For this review, use the dimensioned drawing (mm, ordinates from the lowest corner) and the shaded views. A direction names the side the tool comes from. Coordinates: 2 decimals unless noted, no trailing zeros. Order: outer loops, then holes, each group sorted by start corner. A loop starts at its lowest first (then second) coordinate and runs counter-clockwise, first axis right, second up. Notation, with made-up numbers: M 72.25,-33 L 79.25,-33 A34 ccw 79.25,3 Z; hole C 67,-25 d10. An arc over 180 degrees is marked long. Answer as CSV lines item,"result". Start each with the question number.
Q1. Consider section B-B on x = 12. Write out the cut boundary in (y, z).
Q2. Consider section A-A on y = 11.5. Write out the cut boundary in (x, z).
Q3. Wall thickness on L1, parallel to Z at x = 142, y = 21; L2, parallel to Y at x = 8, z = 34.5; L3, parallel to X at y = 3.25, z = 57: over which ranges is each line inside the solid? List them lowest first. Write a range as [from, to].
Q4. Consider section C-C on z = 37. Write out the cut boundary in (x, y).
Q5. Machinability: for the marked faces 5 and 6, which of the approach directions +Z, -Z, +X, -X, +Y, -Y give a long, thin tool a straight path to every point of the face, cutting with its end or side? Answer none if there is none.
Q6. For P1, Ø6, axis at x = 99.5, y = 10.5, coming from the -Z side; P2, Ø8, axis at y = 18, z = 32.5, coming from the -X side; P3, Ø8, axis at x = 114, z = 22.5, coming from the +Y side, all flat-tipped, find the tip position at first contact; note any pin that passes through.
Q7. The part is to be moulded in two halves that separate along Z. For the marked faces 1, 2, 3 and 4, say which applies: +Z half, -Z half, draft (parallel to the pull), parting line (faces both ways), or undercut.
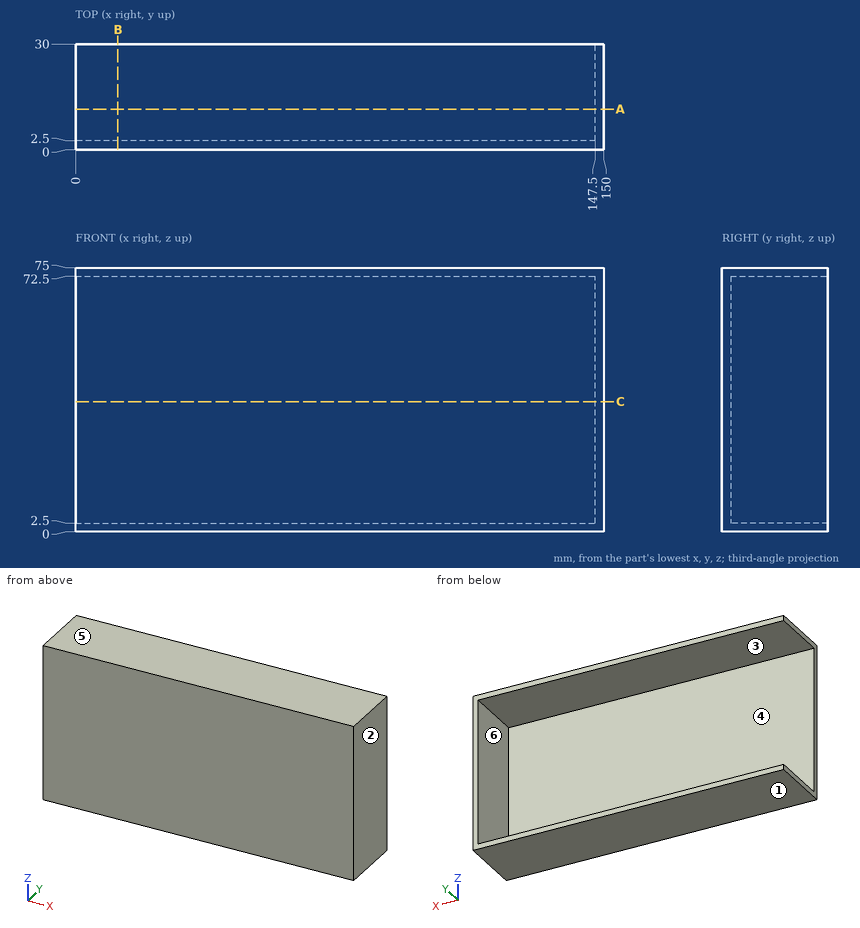
Evaluation:
1,outline,"M 0,0 L 30,0 L 30,2.5 L 2.5,2.5 L 2.5,72.5 L 30,72.5 L 30,75 L 0,75 Z"
2,outline,"M 0,0 L 150,0 L 150,75 L 0,75 L 0,72.5 L 147.5,72.5 L 147.5,2.5 L 0,2.5 Z"
3,L1,"z = [0, 2.5], [72.5, 75]"
3,L2,"y = [0, 2.5]"
3,L3,"x = [147.5, 150]"
4,outline,"M 0,0 L 150,0 L 150,30 L 147.5,30 L 147.5,2.5 L 0,2.5 Z"
5,face 5,"+Z, +X, -X, +Y, -Y"
5,face 6,"-X, +Y"
6,P1,"stops at z = 0"
6,P2,"stops at x = 147.5"
6,P3,"stops at y = 2.5"
7,face 1,"-Z half"
7,face 2,"draft"
7,face 3,"undercut"
7,face 4,"undercut"
